Can you work these out from the model? Positions are in its coordinate system, mm. Face numbers are marked on the shaded views. A direction names the side the tool comes from. Coordinates: 2 decimals unless noted, no trailing zeros. Loops run counter-clockwise (first coordinate to the right, second up) from the corner with the lowest first, then second, coordinate; pieces in that order, holes last. Notation, with made-up numbers: M -2.75,44.25 L 20.25,44.25 A8 ccw 20.25,48.25 Z; hole C 13,19 d11. An arc over 180 degrees is marked long. Return JSON: item names as keys, results as strings. Group by question number.
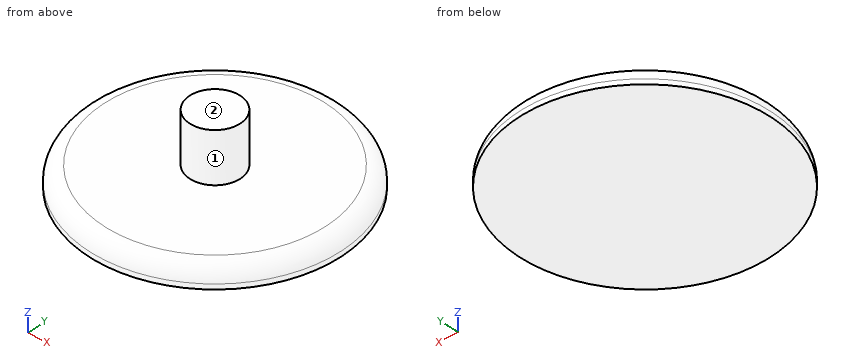
```python
from build123d import *

# Parameters (mm, degrees)
SKETCH_R     = 125
PAD_DEPTH    = 20
SKETCH001_R  = 25
PAD001_DEPTH = 50
FILLET006_R  = 15


with BuildPart() as part:
    # Sketch → Pad (new body)
    with BuildSketch(Plane.XY):
        Circle(SKETCH_R)
    extrude(amount=PAD_DEPTH)

    # Sketch001 (on Face3 of Pad) → Pad001 (join)
    with BuildSketch(Plane.XY.offset(20)):
        Circle(SKETCH001_R)
    extrude(amount=PAD001_DEPTH)

    # Fillet006
    fillet006_edges = [part.edges().sort_by_distance(p)[0] for p in [
        (-125, 0, 20),
    ]]
    fillet(fillet006_edges, radius=FILLET006_R)


solid = part.part
```
1) Suppose I cut it at A-A, the plane x = 0. List the corners of the cut face in (y, z) for me, then the cut area to 3 significant figures.
2) If I drill on line 1 (Z direction, x = -60, y = 71.5); line 2 (Y direction, x = 53.5, z = 9.5); line 3 (X direction, y = 103.5, z = 13), over which ranges is the centre line in solid material (lowest first)? Write a range as from..to.
3) Suppose I cut it at C-C, the plane z = 37. List the corners of the cut face in (x, y) for me.
4) Suppose I cut it at D-D, the plane z = 13.5. List the corners of the cut face in (x, y) for me, then the cut area to 3 significant figures.
5) For pin 1 (1 mm diameter, centred on x = 10.5, z = 51.5, fed in from +Y); pin 2 (4 mm diameter, centred on x = 32, z = 20, fed in from +Y); pin 3 (2 mm diameter, centred on x = 54.5, y = -48.5, fed in from +Z), each with a flat end and sliding along its axis, tell me the tip position at first contact or that it passes through.
6) For the marked faces 1 and 2, which set-ups out of +Z, -Z, +X, -X, +Y, -Y let a thin tool reach every point of the face, with its end or its side?
Returned:
{
 "1": {"outline": "M -125,0 L 125,0 L 125,5 A15 ccw 110,20 L 25,20 L 25,70 L -25,70 L -25,20 L -110,20 A15 ccw -125,5 Z", "area": "7,400 mm²"},
 "2": {"line 1": "z = 0..20", "line 2": "y = -112.21..112.21", "line 3": "x = -65.88..65.88"},
 "3": {"outline": "C 0,0 d50"},
 "4": {"outline": "C 0,0 d244.72", "area": "47,000 mm²"},
 "5": {"pin 1": "stops at y = 22.91", "pin 2": "stops at y = 113.08", "pin 3": "stops at z = 20"},
 "6": {"face 1": "+Z", "face 2": "+Z, +X, -X, +Y, -Y"}
}
